Here's how the part is built. I have some questions about the finished solid (model axes, mm). Face numbers are marked on the shaded views. A direction names the side the tool comes from. Coordinates: 2 decimals unless noted, no trailing zeros. Write each loop counter-clockwise with the first axis right and the second up, starting at its lowest first coordinate (ties: lowest second). Pieces come first, ordered by that corner, then holes. Notation, with made-up numbers: M 44,-34.75 L 100,-34.75 A29 cw 100,1.25 Z; hole C 12.5,18.5 d2. An arc over 180 degrees is marked long. Use one line per item in the form item = value. Start each with the question number.
1. Thinking about a two-plate mould opening in Y: for the marked faces 4, 5 and 6, which applies, released by +Y, released by -Y, zero draft, split by the parting line, or undercut?
2. I want a section at D-D, the plane x = 1. List the corners of the cut face in (y, z) for me.
3. I'm going to push flat-ended pins straight in: pin 1 Ø5.5 at (y, z) = (-9.5, 1.5) entering from -X; pin 2 Ø2 at (y, z) = (14.5, 3) entering from +X; pin 3 Ø10 at (x, y) = (5, -23) entering from +Z. Where does each tip first touch, or does it pass through?
4. I want a section at B-B, the plane z = 2.5. List the corners of the cut face in (x, y) for me.
5. On a 3-axis mill with a long thin cutter (end or side, diameter ignored), from which of +Z, -Z, +X, -X, +Y, -Y can I reach the whole of each face in a straight line? I mean the marked faces 1, 2 and 3. Say none if no direction works.
6. I want a section at A-A, the plane x = 22. List the corners of the cut face in (y, z) for me.
7. I want a section at C-C, the plane y = 11.5. List the corners of the cut face in (x, z) for me, plus the area to 3 significant figures.
8. Please list where these lines run through material, in increasing order: line 1 along Z through (x, y) = (5, -4.5); line 2 along X through (y, z) = (-11.5, 3); line 3 along X through (y, z) = (-22.5, 1). Write a range as [from, to].
from build123d import *

# Parameters (mm, degrees)
F1_DEPTH = 5
F3_DEPTH = 5.1
F4_R     = 1.5
F5_DEPTH = 8
F6_R     = 6
F7_DEPTH = 25


with BuildPart() as f1:
    # F0 (on Top) → F1 (new body)
    with BuildSketch(Plane.XY):
        with BuildLine():
            Line((24.302487, 12.771593), (16.494151, 12.771593))
            ThreePointArc((16.494151, 12.771593), (-6.025428, 22.099508), (3.302487, -0.420071))
            Line((3.302487, -0.420071), (3.302487, -13.292416))
            Line((3.302487, -13.292416), (3.302487, -22.228407))
            Line((3.302487, -22.228407), (12.669307, -22.228407))
            Line((12.669307, -22.228407), (24.302487, -22.228407))
            Line((24.302487, -22.228407), (24.302487, 12.771593))
        make_face()
        Polygon((3.302487, -22.228407), (3.302487, -13.292416), (-0.130287, -12.969643), (-6.076606, -19.139513), (-4.960277, -27.635384), (2.378083, -32.059691), (10.412538, -29.080841), (12.669307, -22.228407), align=None)
    extrude(amount=F1_DEPTH)

    # F2 (on face) → F3 (join)
    with BuildSketch(Plane.XY.offset(5)):
        with BuildLine():
            ThreePointArc((3.302487, -0.420071), (-2.989457, 19.063537), (16.494151, 12.771593))
            ThreePointArc((16.494151, 12.771593), (-6.025428, 22.099508), (3.302487, -0.420071))
        make_face()
    extrude(amount=F3_DEPTH)

    # F4 (on face) → F5 (cut)
    with BuildSketch(Plane.YZ.offset(24.302487)):
        with Locations((-4.728407, 2.5)):
            Circle(F4_R)
    extrude(amount=-F5_DEPTH, mode=Mode.SUBTRACT)

    # F6 (on face) → F7 (cut)
    with BuildSketch(Plane.XY.offset(5)):
        with Locations((3.302487, -23.465436)):
            Circle(F6_R)
    extrude(amount=-F7_DEPTH, mode=Mode.SUBTRACT)


solid = f1.part
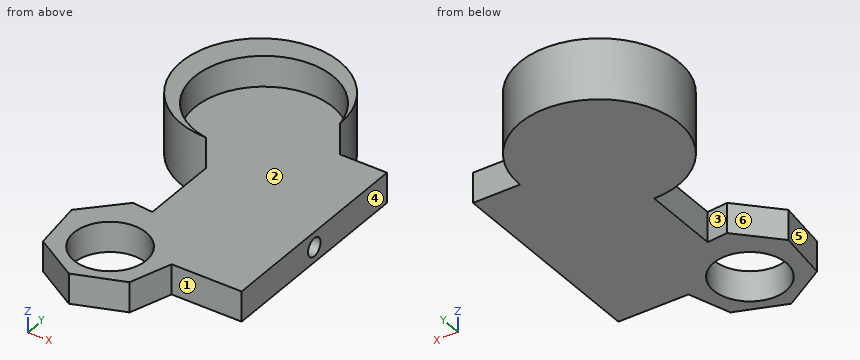
Answer list:
q1.face_4 = zero draft
q1.face_5 = released by -Y
q1.face_6 = undercut
q2.outline = M -31.23,0 L -29.01,0 L -29.01,5 L -31.23,5 Z; M -17.92,0 L -13.08,0 L -13.08,5 L -17.92,5 Z; M -0.22,0 L 25.76,0 L 25.76,10.1 L 21.66,10.1 L 21.66,5 L 0.2,5 L 0.2,10.1 L -0.22,10.1 Z
q3.pin_1 = 3.3
q3.pin_2 = 16.47
q3.pin_3 = 5
q4.outline = M -6.08,-19.14 L -4.96,-27.64 L 2.38,-32.06 L 10.41,-29.08 L 12.67,-22.23 L 24.3,-22.23 L 24.3,-6.23 L 16.3,-6.23 L 16.3,-3.23 L 24.3,-3.23 L 24.3,12.77 L 16.49,12.77 A13.19 ccw long 3.3,-0.42 L 3.3,-13.29 L -0.13,-12.97 Z; hole C 3.3,-23.47 d12
q5.face_1 = +Z, -Z, +X, -Y
q5.face_2 = +Z
q5.face_3 = +Z, -Z
q6.outline = M -22.23,0 L 12.77,0 L 12.77,5 L -22.23,5 Z; hole C -4.73,2.5 d3
q7.outline = M -9.83,0 L 24.3,0 L 24.3,5 L -6.34,5 L -6.34,10.1 L -9.83,10.1 Z
q7.area = 188 mm²
q8.line_1 = [0, 5]
q8.line_2 = [3.3, 24.3]
q8.line_3 = [-5.64, -2.62], [9.22, 12.58]
